Verification items for the finished model (mm, model axes). A direction names the side the tool comes from. Coordinates: 2 decimals unless noted, no trailing zeros. Loops run counter-clockwise (first coordinate to the right, second up) from the corner with the lowest first, then second, coordinate; pieces in that order, holes last. Notation, with made-up numbers: (-25, 21.5) -> (-15, 21.5) arc R18 cw to (-15, 48.5) -> close; hole circle Ø4 at (-23, 40). An arc over 180 degrees is marked (long way). Write item = value, one per line.
Autodesk Inventor part; units mm, degrees
ref_plane "YZ Plane" through (0, 0, 0) normal (1, 0, 0) x (0, 1, 0)
ref_plane "XZ Plane" through (0, 0, 0) normal (0, 1, 0) x (-1, 0, 0)
ref_plane "XY Plane" through (0, 0, 0) normal (0, 0, 1) x (1, 0, 0)
sketch "main" plane through (0, 0, 0) normal (0, 0, 1) x (1, 0, 0)
  line L0 (-3.1973, -8.3156) -> (0.4095, -8.3156)
  arc A0 (-3.1973, -8.3156) -> (-3.7053, -8.8236) centre (-3.1973, -8.8236) ccw
  arc A1 (0.9175, -8.8236) -> (0.4095, -8.3156) centre (0.4095, -8.8236) ccw
  line L1 (-3.7053, -12.4304) -> (-3.7053, -8.8236)
  line L2 (0.9175, -8.8236) -> (0.9175, -12.4304)
  arc A2 (-3.7053, -12.4304) -> (-3.1973, -12.9384) centre (-3.1973, -12.4304) ccw
  line L3 (0.4095, -12.9384) -> (-3.1973, -12.9384)
  arc A3 (0.4095, -12.9384) -> (0.9175, -12.4304) centre (0.4095, -12.4304) ccw
  spline S0 degree 3 poles (4.1061, -10.627) (4.0635, -11.3826) (3.9418, -12.8881) (2.5369, -15.0176) (0.7715, -15.9468) (-0.3245, -16.1781) (-0.6942, -16.259) knots 0 0 0 0 0.294694 0.589389 0.884083 1.03143 1.03143 1.03143 1.03143
  arc A4 (-10.9164, -7.5728) -> (-6.8939, -2.275) centre (-12.3939, -2.275) ccw
  line L4 (-14.5376, -20.1198) -> (-0.6942, -16.259)
  line L5 (-10.9164, -7.5728) -> (-17.5138, -9.5303)
  arc A5 (-17.5138, -9.5303) -> (-14.5376, -20.1198) centre (-16.0578, -14.834) ccw
  circle A6 centre (-16.0578, -14.834) radius 2.1
  line L6 (0.4095, -0.2384) -> (-3.1973, -0.2384)
  arc A7 (-3.7053, 0.2696) -> (-3.1973, -0.2384) centre (-3.1973, 0.2696) ccw
  line L7 (0.9175, 3.8764) -> (0.9175, 0.2696)
  line L8 (-3.7053, 0.2696) -> (-3.7053, 3.8764)
  line L9 (-3.1973, 4.3844) -> (0.4095, 4.3844)
  arc A8 (-3.1973, 4.3844) -> (-3.7053, 3.8764) centre (-3.1973, 3.8764) ccw
  arc A9 (0.9175, 3.8764) -> (0.4095, 4.3844) centre (0.4095, 3.8764) ccw
  arc A10 (0.4095, -0.2384) -> (0.9175, 0.2696) centre (0.4095, 0.2696) ccw
  line L10 (4.1061, -10.627) -> (4.1061, 14.773)
  arc A11 (4.1061, 14.773) -> (-6.8939, 14.773) centre (-1.3939, 14.773) ccw
  line L11 (-6.8939, 14.773) -> (-6.8939, -2.275)
  line L12 (0.4095, 12.4616) -> (-3.1973, 12.4616)
  arc A12 (0.4095, 12.4616) -> (0.9175, 12.9696) centre (0.4095, 12.9696) ccw
  arc A13 (-3.7053, 12.9696) -> (-3.1973, 12.4616) centre (-3.1973, 12.9696) ccw
  line L13 (0.9175, 16.5764) -> (0.9175, 12.9696)
  line L14 (-3.7053, 12.9696) -> (-3.7053, 16.5764)
  arc A14 (-3.1973, 17.0844) -> (-3.7053, 16.5764) centre (-3.1973, 16.5764) ccw
  arc A15 (0.9175, 16.5764) -> (0.4095, 17.0844) centre (0.4095, 16.5764) ccw
  line L15 (-3.1973, 17.0844) -> (0.4095, 17.0844)
  line L16 (-15.2156, -14.4817) -> (-14.3027, -14.4817) construction
  point P0 (-2.9609, 0.4438)
  point P1 (-20.5005, 14.8552)
  dimension "d8" = 5.5
sketch "Sketch1" plane through (0, 0, 0) normal (0, 1, 0) x (-1, 0, 0)
  line L0 (-1.8034, -23.0886) -> (1.8034, -23.0886)
  arc A0 (-1.8034, -23.0886) -> (-2.3114, -23.5966) centre (-1.8034, -23.5966) ccw
  arc A1 (2.3114, -23.5966) -> (1.8034, -23.0886) centre (1.8034, -23.5966) ccw
  line L1 (-2.3114, -27.2034) -> (-2.3114, -23.5966)
  line L2 (2.3114, -23.5966) -> (2.3114, -27.2034)
  arc A2 (-2.3114, -27.2034) -> (-1.8034, -27.7114) centre (-1.8034, -27.2034) ccw
  line L3 (1.8034, -27.7114) -> (-1.8034, -27.7114)
  arc A3 (1.8034, -27.7114) -> (2.3114, -27.2034) centre (1.8034, -27.2034) ccw
  spline S0 degree 3 poles (5.5, -25.4) (5.4573, -26.1557) (5.3357, -27.6611) (3.9308, -29.7907) (2.1654, -30.7198) (1.0693, -30.9511) (0.6997, -31.0321) knots 0 0 0 0 0.294694 0.589389 0.884083 1.03143 1.03143 1.03143 1.03143
  arc A4 (-9.5225, -22.3458) -> (-5.5, -17.048) centre (-11, -17.048) ccw
  line L4 (-13.1438, -34.8928) -> (0.6997, -31.0321)
  line L5 (-9.5225, -22.3458) -> (-16.12, -24.3033)
  arc A5 (-16.12, -24.3033) -> (-13.1438, -34.8928) centre (-14.6639, -29.6071) ccw
  circle A6 centre (-14.6639, -29.6071) radius 2.1
  line L6 (1.8034, -15.0114) -> (-1.8034, -15.0114)
  arc A7 (-2.3114, -14.5034) -> (-1.8034, -15.0114) centre (-1.8034, -14.5034) ccw
  line L7 (2.3114, -10.8966) -> (2.3114, -14.5034)
  line L8 (-2.3114, -14.5034) -> (-2.3114, -10.8966)
  line L9 (-1.8034, -10.3886) -> (1.8034, -10.3886)
  arc A8 (-1.8034, -10.3886) -> (-2.3114, -10.8966) centre (-1.8034, -10.8966) ccw
  arc A9 (2.3114, -10.8966) -> (1.8034, -10.3886) centre (1.8034, -10.8966) ccw
  arc A10 (1.8034, -15.0114) -> (2.3114, -14.5034) centre (1.8034, -14.5034) ccw
  line L10 (5.5, -25.4) -> (5.5, 0)
  arc A11 (5.5, 0) -> (-5.5, 0) centre (0, 0) ccw
  line L11 (-5.5, 0) -> (-5.5, -17.048)
  line L12 (1.8034, -2.3114) -> (-1.8034, -2.3114)
  arc A12 (1.8034, -2.3114) -> (2.3114, -1.8034) centre (1.8034, -1.8034) ccw
  arc A13 (-2.3114, -1.8034) -> (-1.8034, -2.3114) centre (-1.8034, -1.8034) ccw
  line L13 (2.3114, 1.8034) -> (2.3114, -1.8034)
  line L14 (-2.3114, -1.8034) -> (-2.3114, 1.8034)
  arc A14 (-1.8034, 2.3114) -> (-2.3114, 1.8034) centre (-1.8034, 1.8034) ccw
  arc A15 (2.3114, 1.8034) -> (1.8034, 2.3114) centre (1.8034, 1.8034) ccw
  line L15 (-1.8034, 2.3114) -> (1.8034, 2.3114)
  line L16 (-13.8217, -29.2547) -> (-12.9088, -29.2547) construction
extrude "Extrusion1" add sketch "Sketch1" along normal blind 1.5875
properties part number "bent_gusset" material "Acetal Resin, White"
1) Material ranges on line 1 (X direction, y = 1.45, z = -1); line 2 (Z direction, x = 1.25, y = 0.4); line 3 (Z direction, x = 16.25, y = 1), recorded low to high.
Ans:
line_1 = -5.5 to -2.31, 2.31 to 5.5
line_2 = -31.58 to -27.71, -23.09 to -15.01, -10.39 to -2.31, 2.31 to 5.36
line_3 = -34.87 to -30.98, -28.23 to -24.34
2) Tool access check on faces 4 (the face through (2.311, 1, -13)), 5 (the face through (-5.5, 1, -13)). Record the directions out of +Z, -Z, +X, -X, +Y, -Y that give a thin tool (end or side, any length) a straight path to the whole face; none if there is none.
Ans:
face_4 = +Y, -Y
face_5 = +Z, -Z, -X, +Y, -Y
3) Depth check by flat-ended pin: pin 1 Ø2 at (x, z) = (7, -2) entering from +Y; pin 2 Ø0.5 at (x, y) = (-0.5, 1) entering from +Z; pin 3 Ø0.8 at (y, z) = (0.5, -13.5) entering from +X; pin 4 Ø0.5 at (x, y) = (0, 0.5) entering from -Z. Enter the tip coordinate at first touch or a pass-through.
Ans:
pin_1 = through
pin_2 = 5.49
pin_3 = 5.5
pin_4 = -31.3
4) Sectioned sample at D-D, the plane y = 0.45. Count the separate pieces of the cut face and the enclosed holes in it, plus the area to 3 significant figures.
Ans:
separate_pieces = 1
enclosed_holes = 4
area = 467 mm2
5) Sectioned sample at A-A, the plane z = -13. Record the cut outline in (x, y), plus the area to 3 significant figures.
Ans:
outline = (-5.5, 0) -> (-2.31, 0) -> (-2.31, 1.59) -> (-5.5, 1.59) -> close; (2.31, 0) -> (5.5, 0) -> (5.5, 1.59) -> (2.31, 1.59) -> close
area = 10.1 mm2
6) Sectioned sample at B-B, the plane x = 0. Record the cut outline in (y, z), plus the area to 3 significant figures.
Ans:
outline = (0, -31.23) -> (1.59, -31.23) -> (1.59, -27.71) -> (0, -27.71) -> close; (0, -23.09) -> (1.59, -23.09) -> (1.59, -15.01) -> (0, -15.01) -> close; (0, -10.39) -> (1.59, -10.39) -> (1.59, -2.31) -> (0, -2.31) -> close; (0, 2.31) -> (1.59, 2.31) -> (1.59, 5.5) -> (0, 5.5) -> close
area = 36.3 mm2
7) Sectioned sample at C-C, the plane z = -25. Record the cut outline in (x, y).
Ans:
outline = (-5.5, 0) -> (-2.31, 0) -> (-2.31, 1.59) -> (-5.5, 1.59) -> close; (2.31, 0) -> (17.67, 0) -> (17.67, 1.59) -> (2.31, 1.59) -> close
8) Release check for a two-part mould opening along Z. For faces 1 (the face through (12.775, 0.783, -23.311)), 2 (the face through (5.5, 1, -8)), 3 (the face through (0, 1, -10.389)) record: pulls with the +Z half, pulls with the -Z half, needs draft (parallel to the pull), parting line crosses it, or undercut.
Ans:
face_1 = pulls with the +Z half
face_2 = needs draft
face_3 = undercut
